Build history of the part. All positions in model axes, mm. A direction names the side the tool comes from. Coordinates: 2 decimals unless noted, no trailing zeros. Order: outer loops, then holes, each group sorted by start corner. A loop starts at its lowest first (then second) coordinate and runs counter-clockwise, first axis right, second up. Notation, with made-up numbers: (26, -35) - (52, -35) arc R25 ccw to (52, -22) - close; hole circle Ø4 at (50.5, 35). An arc over 180 degrees is marked (long way). Return JSON: item names as keys, results as strings.
from build123d import *

# Parameters (mm, degrees)
SKETCH1_R           = 2.475
BOSS_EXTRUDE1_DEPTH = 0.625
SKETCH3_R           = 3.975
BOSS_EXTRUDE2_DEPTH = 1


with BuildPart() as part:
    # Sketch1 → Boss-Extrude1 (new, symmetric)
    with BuildSketch(Plane(origin=(0, 0, 0), x_dir=(1, 0, 0), z_dir=(0, 1, 0))):
        with Locations(Location((0, 0, 0), (0, 0, 270))):
            Circle(SKETCH1_R)
    extrude(amount=BOSS_EXTRUDE1_DEPTH, both=True)

    # Sketch3 → Boss-Extrude2 (add)
    with BuildSketch(Plane(origin=(0, 0.625, 0), x_dir=(1, 0, 0), z_dir=(0, 1, 0))):
        with Locations(Location((0, 0, 0), (0, 0, 270))):
            Circle(SKETCH3_R)
    boss_extrude2 = extrude(amount=BOSS_EXTRUDE2_DEPTH)

    # Mirror1: Boss-Extrude2 across plane
    add(boss_extrude2.mirror(Plane.ZX))


solid = part.part
1. Cut at A-A on z = 0. Give the cut face in (x, y) (3 decimals).
Check values:
{"outline": "(-3.975, -1.625) - (3.975, -1.625) - (3.975, -0.625) - (2.475, -0.625) - (2.475, 0.625) - (3.975, 0.625) - (3.975, 1.625) - (-3.975, 1.625) - (-3.975, 0.625) - (-2.475, 0.625) - (-2.475, -0.625) - (-3.975, -0.625) - close"}
2. Probe L1, parallel to Y at x = -2.5, z = -0.25 (3 decimals); L2, parallel to X at y = -1.4, z = -3.5; L3, parallel to Z at x = 0.75, y = -1. List the from-to ranges inside material, lowest first.
Check values:
{"L1": "-1.625 to -0.625, 0.625 to 1.625", "L2": "-1.88 to 1.88", "L3": "-3.9 to 3.9"}
3. Drop flat-ended pins along their axis: pin 1 (1.5 mm diameter, centred on x = -2, y = -0.5, fed in from -Z); pin 2 (1 mm diameter, centred on y = -0.5, z = 3, fed in from -X); pin 3 (1.5 mm diameter, centred on x = 2.5, y = 0, fed in from -Z). Give the stop position or say it passes through.
Check values:
{"pin 1": "z = -3.77", "pin 2": "x = -3.08", "pin 3": "z = -3.38"}
4. Mould opens along Y. For faces 3 (the cylindrical face through (0.74, 0.01, 2.36)), 4 (the flat face through (0, -1.625, 0)), 5 (the cylindrical face through (-2.419, 1.118, -3.154)) say: pulls with the +Y half, pulls with the -Y half, needs draft (parallel to the pull), parting line crosses it, or undercut.
Check values:
{"face 3": "undercut", "face 4": "pulls with the -Y half", "face 5": "needs draft"}
5. Tool access for faces 1 (the flat face through (-2, 0.625, -2)), 2 (the cylindrical face through (-2.419, -1.118, -3.154)): list every direction of +Z, -Z, +X, -X, +Y, -Y with a clear straight run to the whole face (end or side of a thin tool).
Check values:
{"face 1": "none", "face 2": "+Y, -Y"}
6. Cut at D-D on y = 0. Give the cut face in (x, z) (3 decimals).
Check values:
{"outline": "circle Ø4.95 at (0, 0)"}
7. Cut at C-C on y = -0.75. Give the cut face in (x, z) (3 decimals), plus the area to 3 significant figures.
Check values:
{"outline": "circle Ø7.95 at (0, 0)", "area": "49.6 mm²"}
8. Cut at B-B on x = 0. Give the cut face in (y, z) (3 decimals), plus the area to 3 significant figures.
Check values:
{"outline": "(-1.625, -3.975) - (-0.625, -3.975) - (-0.625, -2.475) - (0.625, -2.475) - (0.625, -3.975) - (1.625, -3.975) - (1.625, 3.975) - (0.625, 3.975) - (0.625, 2.475) - (-0.625, 2.475) - (-0.625, 3.975) - (-1.625, 3.975) - close", "area": "22.1 mm²"}
